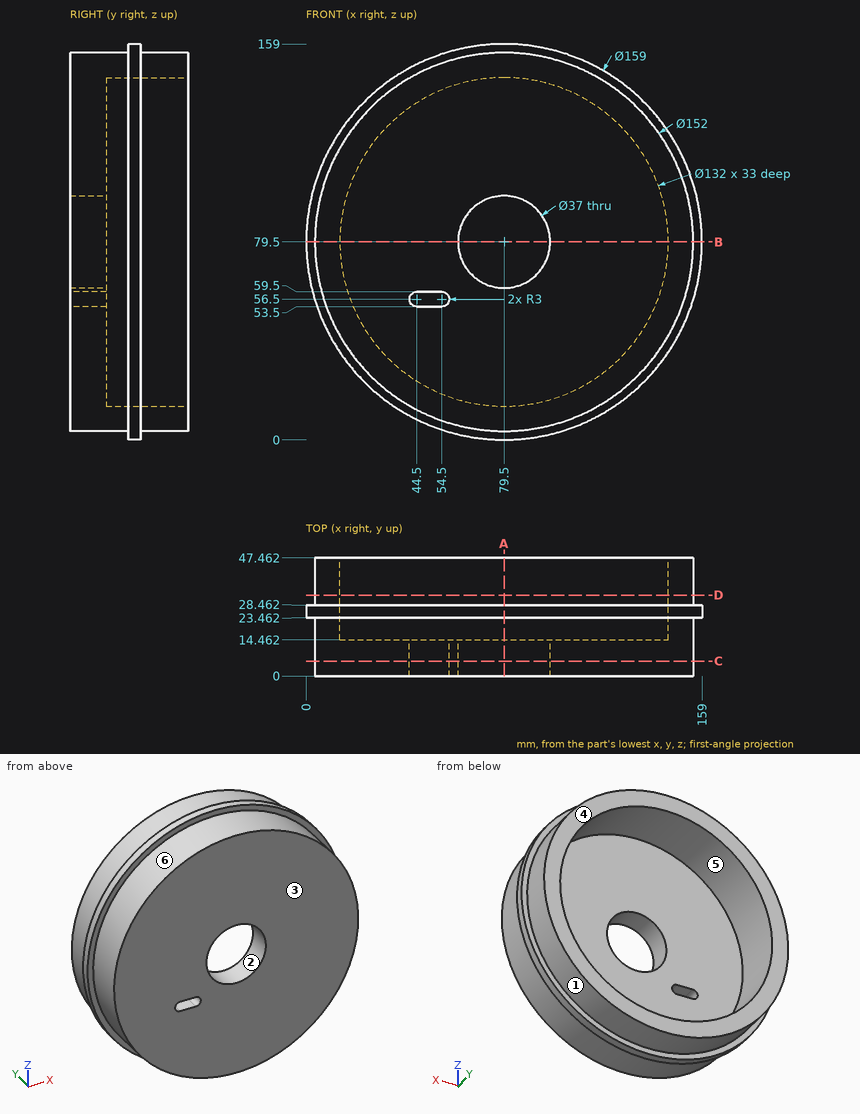
Design review of the part shown in the three views and the two pictorial views. Dimensions are in mm from the part's minimum x, y and z. A direction names the side the tool comes from. Round coordinates to 2 decimals unless told otherwise and drop trailing zeros. Loops run counter-clockwise (first coordinate to the right, second up) from the corner with the lowest first, then second, coordinate; pieces in that order, holes last. Notation, with made-up numbers: (15, -10.5) -> (58, -10.5) arc R25 cw to (58, 25.5) -> close; hole circle Ø7 at (17.5, 14.25). An arc over 180 degrees is marked (long way). Return JSON: item names as keys, results as strings.
(1) For line 1 (X direction, y = 11, z = 79); line 2 (Y direction, x = 88, z = 98); line 3 (Z direction, x = 79, y = 35), list the stretches that pass through material, from the lowest coordinate up.
Solved:
{"line 1": "3.5 to 61.01, 97.99 to 155.5", "line 2": "0 to 14.46", "line 3": "3.5 to 13.5, 145.5 to 155.5"}
(2) Add section D-D on y = 32.5. Write out the cut boundary in (x, z), plus the area to 3 significant figures.
Solved:
{"outline": "circle Ø152 at (79.5, 79.5); hole circle Ø132 at (79.5, 79.5)", "area": "4,460 mm2"}
(3) Add section C-C on y = 6. Write out the cut boundary in (x, z).
Solved:
{"outline": "circle Ø152 at (79.5, 79.5); hole (44.5, 53.5) -> (54.5, 53.5) arc R3 ccw to (54.5, 59.5) -> (44.5, 59.5) arc R3 ccw to start; hole circle Ø37 at (79.5, 79.5)"}
(4) Add section B-B on z = 79.5. Write out the cut boundary in (x, y), plus the area to 3 significant figures.
Solved:
{"outline": "(0, 23.46) -> (3.5, 23.46) -> (3.5, 0) -> (61, 0) -> (61, 14.46) -> (13.5, 14.46) -> (13.5, 47.46) -> (3.5, 47.46) -> (3.5, 28.46) -> (0, 28.46) -> close; (98, 0) -> (155.5, 0) -> (155.5, 23.46) -> (159, 23.46) -> (159, 28.46) -> (155.5, 28.46) -> (155.5, 47.46) -> (145.5, 47.46) -> (145.5, 14.46) -> (98, 14.46) -> close", "area": "2,360 mm2"}
(5) The part is to be moulded in two halves that separate along X. For the marked faces 1, 2 and 3, say which applies: released by +X, released by -X, zero draft, split by the parting line, or undercut.
Solved:
{"face 1": "split by the parting line", "face 2": "undercut", "face 3": "zero draft"}
(6) For the marked faces 4, 5 and 6, list the 3-axis set-ups (+Z, -Z, +X, -X, +Y, -Y) from which the entire face can be reached by the end or side of a thin tool; tool diameter is ignored.
Solved:
{"face 4": "+Z, -Z, +X, -X, +Y", "face 5": "+Y", "face 6": "-Y"}
(7) For pin 1 (6 mm diameter, centred on y = 24.5, z = 137, fed in from -X); pin 2 (12 mm diameter, centred on x = 142.5, y = 20.5, fed in from +Z) (1 decimal); pin 3 (1.5 mm diameter, centred on x = 100, y = 34, fed in from -Z), all flat-tipped, find the tip position at first contact; note any pin that passes through.
Solved:
{"pin 1": "x = 21.62", "pin 2": "z = 134.1", "pin 3": "z = 6.11"}
(8) Add section A-A on x = 79.5. Write out the cut boundary in (y, z), plus the area to 3 significant figures.
Solved:
{"outline": "(0, 3.5) -> (23.46, 3.5) -> (23.46, 0) -> (28.46, 0) -> (28.46, 3.5) -> (47.46, 3.5) -> (47.46, 13.5) -> (14.46, 13.5) -> (14.46, 61) -> (0, 61) -> close; (0, 98) -> (14.46, 98) -> (14.46, 145.5) -> (47.46, 145.5) -> (47.46, 155.5) -> (28.46, 155.5) -> (28.46, 159) -> (23.46, 159) -> (23.46, 155.5) -> (0, 155.5) -> close", "area": "2,360 mm2"}
